The listing builds one solid part. Answer for the finished solid, in the listing's coordinates (mm). Face numbers are marked on the shaded views. A direction names the side the tool comes from. Give positions to 0.01 mm unless a question says otherwise; leave off trailing zeros. Loops run counter-clockwise (first coordinate to the right, second up) from the corner with the lowest first, then second, coordinate; pieces in that order, holes last. Notation, with made-up numbers: M 1,30 L 9,30 A36 cw 9,64 Z; hole C 64,15 d8. An arc over 180 degrees is marked long. One line per item, written item: value. Start each with the question number.
Q1. For the marked faces 4 and 5, determine the directions among +Z, -Z, +X, -X, +Y, -Y from which every point of the face is accessible in a straight line to the end or side of a thin tool.
Q2. A cutting plane is placed at B-B, the plane x = -68.5. Determine the outline of the cut face in (y, z).
Q3. A cutting plane is placed at A-A, the plane x = 0. Determine the outline of the cut face in (y, z), and give its area (4 significant figures).
Q4. Flat-ended cylindrical pins translate along their axes: pin 1 (24 mm diameter, centred on x = -55, y = -80, fed in from -Z); pin 2 (2 mm diameter, centred on y = -0.5, z = 1, fed in from +X); pin 3 (0.8 mm diameter, centred on y = 11.5, z = 7, fed in from +X); pin 4 (5 mm diameter, centred on x = 8.5, z = 3, fed in from +Y). Find the tip coordinate at first contact, or state that the pin passes through.
Q5. Consider L1, parallel to Y at x = 0, z = 4.25; L2, parallel to X at y = -65.5, z = 8.5; L3, parallel to Y at x = 43, z = 8.25. Determine where each line is inside the solid, lowest interval first.
Q6. A cutting plane is placed at C-C, the plane y = -77. Determine the outline of the cut face in (x, z).
Q7. The mould has two halves that part along X. Classify the marked faces 1, 2 and 3: +X half, -X half, draft (parallel to the pull), parting line (faces both ways), or undercut.
Q8. A cutting plane is placed at D-D, the plane z = 5.75. State how many separate pieces and enclosed holes the cut face has, and give its area (3 significant figures).
from build123d import *

# Parameters (mm, degrees)
F1_R            = 20
F2_DEPTH        = 10
F3_T            = -5
F4_DEPTH        = 5.001
F1_R_2          = 4.15
F5_DEPTH        = 10
F6_DEPTH        = 10
F6_COPIES_COUNT = 3
F9_R            = 5
F10_T1_DEPTH    = 10
F11_R           = 5


# Not quite as in the source:
# - a fillet or chamfer that OpenCascade refuses, or shapes differently, is made with other operations: its cross-section is extruded or revolved along the edge and cut away or added
# - a feature of the source that left no trace in its solid (it failed there, or was rolled back) is left out
# - a pattern or mirror of a feature is missing from the dataset's text; its kind, count and spacing are read off the source's solid


with BuildPart() as f2:
    # F1 (on Top) → F2 (new body)
    with BuildSketch(Plane.XY):
        with BuildLine():
            ThreePointArc((-25, 0), (0, -25), (25, 0))
            ThreePointArc((25, 0), (0, 25), (-25, 0))
        make_face()
        with BuildLine():
            ThreePointArc((3.5, 19.6913686675), (15.3297097168, 12.8452325787), (20, 0))
            ThreePointArc((20, 0), (-12.8452325787, -15.3297097168), (-3.5, 19.6913686675))
            ThreePointArc((-3.5, 19.6913686675), (0, 20), (3.5, 19.6913686675))
        make_face(mode=Mode.SUBTRACT)
        with BuildLine():
            ThreePointArc((55, -55), (33.982083659, -30.7824998224), (25, 0))
            ThreePointArc((25, 0), (0, -25), (-25, 0))
            ThreePointArc((-25, 0), (-33.982083659, -30.7824998224), (-55, -55))
            ThreePointArc((-55, -55), (-37.3223304703, -62.3223304703), (-30, -80))
            ThreePointArc((-30, -80), (-37.3223304703, -97.6776695297), (-55, -105))
            Line((-55, -105), (55, -105))
            ThreePointArc((55, -105), (30, -80), (55, -55))
        make_face()
        with BuildLine():
            ThreePointArc((80, -80), (72.6776695297, -62.3223304703), (55, -55))
            ThreePointArc((55, -55), (30, -80), (55, -105))
            ThreePointArc((55, -105), (72.6776695297, -97.6776695297), (80, -80))
        make_face()
        with Locations((55, -80)):
            Circle(F1_R, mode=Mode.SUBTRACT)
        with BuildLine():
            ThreePointArc((-30, -80), (-37.3223304703, -62.3223304703), (-55, -55))
            ThreePointArc((-55, -55), (-80, -80), (-55, -105))
            ThreePointArc((-55, -105), (-37.3223304703, -97.6776695297), (-30, -80))
        make_face()
        with Locations((-55, -80)):
            Circle(F1_R, mode=Mode.SUBTRACT)
    extrude(amount=F2_DEPTH)

    # F3
    f3_openings = [f2.faces().sort_by_distance(p)[0] for p in [
        (0, -59.438768, 10),
    ]]
    offset(amount=F3_T, openings=f3_openings)

    # F4 (cut, through all): a face of the model
    f4_faces = [f2.faces().sort_by_distance(p)[0] for p in [
        (0, -60.9945168835, 5),
    ]]
    extrude(f4_faces, amount=-F4_DEPTH, mode=Mode.SUBTRACT)



with BuildPart() as f5:
    # F1 (on Top) → F5 (new body, through all)
    with BuildSketch(Plane.XY):
        with BuildLine():
            ThreePointArc((9.15, 0), (7.6074798718, 5.0841665984), (3.5, 8.4541409972))
            ThreePointArc((3.5, 8.4541409972), (0, 9.15), (-3.5, 8.4541409972))
            ThreePointArc((-3.5, 8.4541409972), (-5.0841665984, -7.6074798718), (9.15, 0))
        make_face()
        Circle(F1_R_2, mode=Mode.SUBTRACT)
    extrude(amount=F5_DEPTH)


with BuildPart() as f2_1:
    add(f2.part)

    add(f5.part)  # F6 merges F5
    # F1 (on Top) → F6 (join, through all)
    with BuildSketch(Plane.XY):
        with BuildLine():
            Line((3.5, 8.4541409972), (3.5, 19.6913686675))
            ThreePointArc((3.5, 19.6913686675), (0, 20), (-3.5, 19.6913686675))
            Line((-3.5, 19.6913686675), (-3.5, 8.4541409972))
            ThreePointArc((-3.5, 8.4541409972), (0, 9.15), (3.5, 8.4541409972))
        make_face()
    f6 = extrude(amount=F6_DEPTH)

    # F6_copies: F6 ×3 about axis
    f6_copies_axis = Axis((0, 0, 0), (0, 0, 1))
    for i in range(1, F6_COPIES_COUNT):
        add(f6.rotate(f6_copies_axis, i * 360 / F6_COPIES_COUNT))

    # F9
    f9_edges = [f2_1.edges().sort_by_distance(p)[0] for p in [
        (3.5, 8.454141, 5),
        (3.5, 19.691369, 5),
        (-3.5, 8.454141, 5),
        (-3.5, 19.691369, 5),
    ]]
    fillet(f9_edges, radius=F9_R)

    # F10: fillet of radius 10 on 4 edges, made by hand

    # F10_s2 → F10_t1 (join)
    with BuildSketch(Plane.XY):
        with BuildLine():
            ThreePointArc((57.6335213289, -55.1390956438), (54.8351268274, -54.4231472749), (52.358111127, -52.9372175751))
            ThreePointArc((52.358111127, -52.9372175751), (53.6675306909, -53.9833691579), (55, -55))
            ThreePointArc((55, -55), (56.3185960515, -55.0347981291), (57.6335213289, -55.1390956438))
        make_face()
        with BuildLine():
            ThreePointArc((-52.358111127, -52.9372175751), (-54.8351268274, -54.4231472749), (-57.6335213289, -55.1390956438))
            ThreePointArc((-57.6335213289, -55.1390956438), (-56.3185960515, -55.0347981291), (-55, -55))
            ThreePointArc((-55, -55), (-53.6675306909, -53.9833691579), (-52.358111127, -52.9372175751))
        make_face()
        with BuildLine():
            ThreePointArc((-24.9985005196, 0.2738097395), (-25.0067330939, -0.0368678872), (-25.0246159735, -0.3471396482))
            ThreePointArc((-25.0246159735, -0.3471396482), (-25.0121066389, -0.1735841019), (-25, 0))
            ThreePointArc((-25, 0), (-24.9996251271, 0.1369069227), (-24.9985005196, 0.2738097395))
        make_face()
        with BuildLine():
            ThreePointArc((24.9985005196, 0.2738097395), (25.0067330939, -0.0368678872), (25.0246159735, -0.3471396482))
            ThreePointArc((25.0246159735, -0.3471396482), (25.0121066389, -0.1735841019), (25, 0))
            ThreePointArc((25, 0), (24.9996251271, 0.1369069227), (24.9985005196, 0.2738097395))
        make_face()
    extrude(amount=F10_T1_DEPTH)

    # F11
    f11_edges = [f2_1.edges().sort_by_distance(p)[0] for p in [
        (9.071501, -1.195982, 5),
        (18.803226, -6.814595, 5),
        (-5.571501, -7.258159, 5),
        (5.571501, -7.258159, 5),
        (15.303226, -12.876773, 5),
        (-15.303226, -12.876773, 5),
        (21.751654, -12.323374, 5),
        (48.164428, -55.952652, 5),
        (40, -100, 5),
        (-40, -100, 5),
        (-48.164428, -55.952652, 5),
        (-21.751654, -12.323374, 5),
        (-9.071501, -1.195982, 5),
        (-18.803226, -6.814595, 5),
    ]]
    fillet(f11_edges, radius=F11_R)


solid = f2_1.part
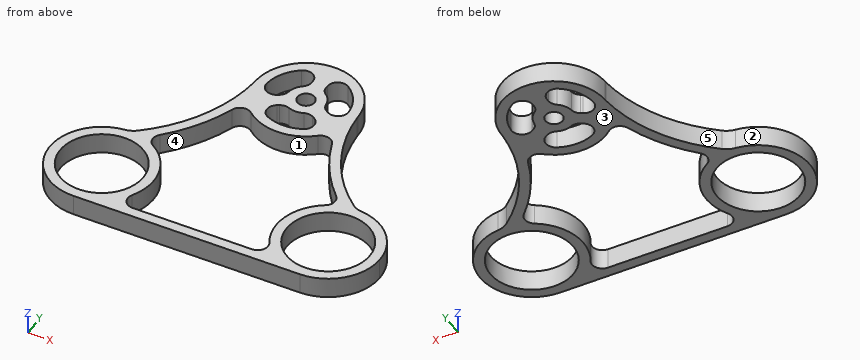
Answer block:
1. face 4: +Z, -Z
1. face 5: +Z, -Z, -X, +Y
2. outline: M -101.04,0 L -94.76,0 L -94.76,10 L -101.04,10 Z; M -65.24,0 L -58.96,0 L -58.96,10 L -65.24,10 Z
3. outline: M -105,0 L -100,0 L -100,10 L -105,10 Z; M -25,0 L -20,0 L -20,10 L -25,10 Z; M -9.15,0 L -4.15,0 L -4.15,10 L -9.15,10 Z; M 4.15,0 L 25,0 L 25,10 L 4.15,10 Z
3. area: 358.5 mm^2
4. pin 1: through
4. pin 2: x = 25.12
4. pin 3: x = 22.4
4. pin 4: y = 24.27
5. L1: -105 to -100, -25 to -20, -9.15 to -4.15, 4.15 to 25
5. L2: -75.37 to -68.77, -41.23 to -34.63, 34.63 to 41.23, 68.77 to 75.37
5. L3: -105 to -96, -64 to -57.76, -51.19 to -43.82
6. outline: M -79.82,0 L -74.77,0 L -74.77,10 L -79.82,10 Z; M -35.23,0 L -30.18,0 L -30.18,10 L -35.23,10 Z; M 30.18,0 L 35.23,0 L 35.23,10 L 30.18,10 Z; M 74.77,0 L 79.82,0 L 79.82,10 L 74.77,10 Z
7. face 1: undercut
7. face 2: -X half
7. face 3: draft
8. separate pieces: 1
8. enclosed holes: 7
8. area: 3,770 mm^2
